```python
from build123d import *

# Parameters (mm, degrees)
SKETCH_1_W               = 100
SKETCH_1_H               = 60
EXTRUDE_1_DEPTH          = 10
SKETCH_2_R               = 5
CUT_EXTRUDE_1_DEPTH      = 20
SKETCH_3_R               = 3
CUT_EXTRUDE_2_DEPTH      = 20
PATTERN_CIRCULAR_1_COUNT = 4


with BuildPart() as part:
    # 草图1 → 凸台-拉伸1 (new body)
    with BuildSketch(Plane(origin=(0, 0, 0), x_dir=(1, 0, 0), z_dir=(0, 1, 0))):
        Rectangle(SKETCH_1_W, SKETCH_1_H)
    extrude(amount=EXTRUDE_1_DEPTH)

    # 草图2 → 切除-拉伸1 (cut)
    with BuildSketch(Plane(origin=(0, 0, 0), x_dir=(1, 0, 0), z_dir=(0, 1, 0))):
        with Locations(Location((0, 0, 0), (0, 0, 90))):
            Circle(SKETCH_2_R)
    extrude(amount=CUT_EXTRUDE_1_DEPTH, mode=Mode.SUBTRACT)

    # 草图3 → 切除-拉伸2 (cut)
    with BuildSketch(Plane(origin=(0, 0, 0), x_dir=(1, 0, 0), z_dir=(0, 1, 0))):
        with Locations(Location((20, 0, 0), (0, 0, 90))):
            Circle(SKETCH_3_R)
    cut_extrude_2 = extrude(amount=CUT_EXTRUDE_2_DEPTH, mode=Mode.SUBTRACT)

    # 阵列(圆周)1: 切除-拉伸2 ×4 about axis
    pattern_circular_1_axis = Axis((0, 0, 0), (0, 1, 0))
    for i in range(1, PATTERN_CIRCULAR_1_COUNT):
        add(cut_extrude_2.rotate(pattern_circular_1_axis, i * 360 / PATTERN_CIRCULAR_1_COUNT), mode=Mode.SUBTRACT)


solid = part.part
```
Verification items for the finished model (mm, model axes). Coordinates: 2 decimals unless noted, no trailing zeros. Loops run counter-clockwise (first coordinate to the right, second up) from the corner with the lowest first, then second, coordinate; pieces in that order, holes last. Notation, with made-up numbers: (28, 64) - (55, 64) arc R16 ccw to (55, 88) - close; hole circle Ø5 at (-6, 6.5). An arc over 180 degrees is marked (long way). Put each result on its own line as item: value.
Item 1: Section check C-C (x = 0). Enter the section's corners in (y, z).
Conclusion:
outline: (0, -30) - (10, -30) - (10, -23) - (0, -23) - close; (0, -17) - (10, -17) - (10, -5) - (0, -5) - close; (0, 5) - (10, 5) - (10, 17) - (0, 17) - close; (0, 23) - (10, 23) - (10, 30) - (0, 30) - close
Item 2: Gauge pin test, flat end, axial feed: pin 1 Ø9 at (x, z) = (0, 0) entering from -Y. Record the tip position at first contact, or that the pin passes through.
Conclusion:
pin 1: passes through
Item 3: Section check B-B (x = 20). Enter the section's corners in (y, z).
Conclusion:
outline: (0, -30) - (10, -30) - (10, -3) - (0, -3) - close; (0, 3) - (10, 3) - (10, 30) - (0, 30) - close
Item 4: Draft check along X on faces 1 (the face through (-50, 5, 0)), 2 (the face through (4.88, 4.93, 1.08)), 3 (the face through (50, 5, 0)). Enter one of: pulls with the +X half, pulls with the -X half, needs draft (parallel to the pull), parting line crosses it, or undercut.
Conclusion:
face 1: pulls with the -X half
face 2: undercut
face 3: pulls with the +X half
Item 5: Section check D-D (z = 22). Enter the section's corners in (x, y).
Conclusion:
outline: (-50, 0) - (-2.24, 0) - (-2.24, 10) - (-50, 10) - close; (2.24, 0) - (50, 0) - (50, 10) - (2.24, 10) - close
Item 6: Section check A-A (z = 0). Enter the section's corners in (x, y).
Conclusion:
outline: (-50, 0) - (-23, 0) - (-23, 10) - (-50, 10) - close; (-17, 0) - (-5, 0) - (-5, 10) - (-17, 10) - close; (5, 0) - (17, 0) - (17, 10) - (5, 10) - close; (23, 0) - (50, 0) - (50, 10) - (23, 10) - close
Item 7: Scan lines: line 1 along X through (y, z) = (6.25, 0); line 2 along X through (y, z) = (5.75, -20); line 3 along Z through (x, y) = (20, 2). Record each from-to range of solid material in increasing order.
Conclusion:
line 1: x = -50 to -23, -17 to -5, 5 to 17, 23 to 50
line 2: x = -50 to -3, 3 to 50
line 3: z = -30 to -3, 3 to 30
